```python
from build123d import *

# Parameters (mm, degrees)
SKETCH001_W     = 308.102
SKETCH001_H     = 147.6375
PAD_DEPTH       = 12.7
SKETCH002_W     = 292.1
SKETCH002_H     = 128.5875
POCKET_DEPTH    = 3.556
SKETCH_W        = 300.0375
SKETCH_H        = 134.9375
POCKET001_DEPTH = 1.778
SKETCH003_W     = 20.6375
SKETCH003_H     = 38.1
POCKET002_DEPTH = 7.9375
SKETCH004_W     = 107.95
SKETCH004_H     = 34.925
POCKET003_DEPTH = 3.175


with BuildPart() as part:
    # Sketch001 → Pad (new body)
    with BuildSketch(Plane.XY):
        Rectangle(SKETCH001_W, SKETCH001_H)
    extrude(amount=PAD_DEPTH)

    # Sketch002 → Pocket (cut)
    with BuildSketch(Plane.XY.offset(12.7)):
        Rectangle(SKETCH002_W, SKETCH002_H)
    extrude(amount=-POCKET_DEPTH, mode=Mode.SUBTRACT)

    # Sketch → Pocket001 (cut)
    with BuildSketch(Plane.XY.offset(12.7)):
        Rectangle(SKETCH_W, SKETCH_H)
    extrude(amount=-POCKET001_DEPTH, mode=Mode.SUBTRACT)

    # Sketch003 → Pocket002 (cut)
    with BuildSketch(Plane.XY.offset(10.922)):
        with Locations((0, 48.41875)):
            Rectangle(SKETCH003_W, SKETCH003_H)
    extrude(amount=-POCKET002_DEPTH, mode=Mode.SUBTRACT)

    # Sketch004 → Pocket003 (cut)
    with BuildSketch(Plane.XY.offset(9.144)):
        with Locations((-64.29375, 46.83125)):
            Rectangle(SKETCH004_W, SKETCH004_H)
    extrude(amount=-POCKET003_DEPTH, mode=Mode.SUBTRACT)


solid = part.part
```
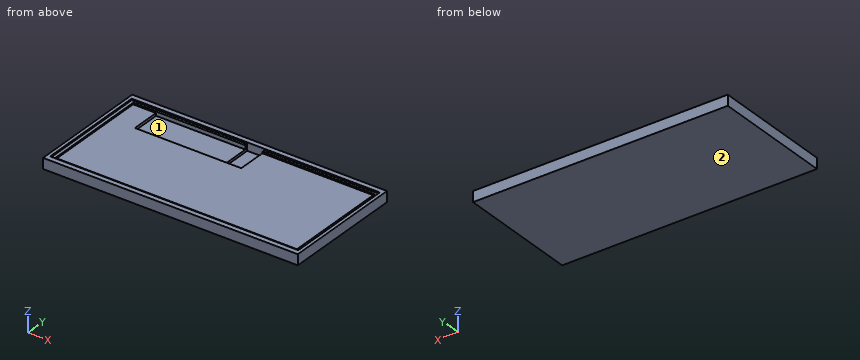
CAD build for the part. Positions are in the model's coordinates, mm. Face numbers are marked on the shaded views. Round coordinates to 2 decimals unless told otherwise and drop trailing zeros. Write each loop counter-clockwise with the first axis right and the second up, starting at its lowest first coordinate (ties: lowest second). Pieces come first, ordered by that corner, then holes. Notation, with made-up numbers: (65, 34) -> (74, 34) arc R11 cw to (74, 54) -> close; hole circle Ø5 at (80, 44.5). An arc over 180 degrees is marked (long way). Answer in a Markdown table with one row per item. Add a question column.
Item 1: Saw through at A-A, the plane x = -4.5. Write the cut outline in (y, z), then the cut area to 3 significant figures.
Item 2: Saw through at D-D, the plane x = -93. Write the cut outline in (y, z), then the cut area to 3 significant figures.
Item 3: Drop flat-ended pins along their axis: pin 1 Ø6 at (x, y) = (40, -8) entering from -Z; pin 2 Ø8 at (x, y) = (-81.5, 11.5) entering from +Z; pin 3 Ø6 at (x, y) = (-2.5, 40) entering from +Z. Give the stop position or say it passes through.
Item 4: Saw through at C-C, the plane x = 109.5. Write the cut outline in (y, z).
Item 5: Drill centre lines: line 1 (X direction, y = -49.5, z = 12.25); line 2 (X direction, y = -31.5, z = 9.75); line 3 (Y direction, x = -88, z = 8.25). Where is each one in solid material? Low to high. Write a range as from..to.
Item 6: Saw through at B-B, the plane y = 38.5. Write the cut outline in (x, z).
Item 7: Mould opens along X. For the marked faces 1 and 2 say: pulls with the +X half, pulls with the -X half, needs draft (parallel to the pull), parting line crosses it, or undercut.
Findings below:
| question | item | result |
|---|---|---|
| 1 | outline | (-73.82, 0) -> (73.82, 0) -> (73.82, 12.7) -> (67.47, 12.7) -> (67.47, 2.98) -> (29.37, 2.98) -> (29.37, 9.14) -> (-64.29, 9.14) -> (-64.29, 10.92) -> (-67.47, 10.92) -> (-67.47, 12.7) -> (-73.82, 12.7) -> close |
| 1 | area | 1,170 mm^2 |
| 2 | outline | (-73.82, 0) -> (73.82, 0) -> (73.82, 12.7) -> (67.47, 12.7) -> (67.47, 10.92) -> (64.29, 10.92) -> (64.29, 5.97) -> (29.37, 5.97) -> (29.37, 9.14) -> (-64.29, 9.14) -> (-64.29, 10.92) -> (-67.47, 10.92) -> (-67.47, 12.7) -> (-73.82, 12.7) -> close |
| 2 | area | 1,300 mm^2 |
| 3 | pin 1 | stops at z = 0 |
| 3 | pin 2 | stops at z = 9.14 |
| 3 | pin 3 | stops at z = 2.98 |
| 4 | outline | (-73.82, 0) -> (73.82, 0) -> (73.82, 12.7) -> (67.47, 12.7) -> (67.47, 10.92) -> (64.29, 10.92) -> (64.29, 9.14) -> (-64.29, 9.14) -> (-64.29, 10.92) -> (-67.47, 10.92) -> (-67.47, 12.7) -> (-73.82, 12.7) -> close |
| 5 | line 1 | x = -154.05..-150.02, 150.02..154.05 |
| 5 | line 2 | x = -154.05..-146.05, 146.05..154.05 |
| 5 | line 3 | y = -73.82..29.37, 64.29..73.82 |
| 6 | outline | (-154.05, 0) -> (154.05, 0) -> (154.05, 12.7) -> (150.02, 12.7) -> (150.02, 10.92) -> (146.05, 10.92) -> (146.05, 9.14) -> (10.32, 9.14) -> (10.32, 2.98) -> (-10.32, 2.98) -> (-10.32, 5.97) -> (-118.27, 5.97) -> (-118.27, 9.14) -> (-146.05, 9.14) -> (-146.05, 10.92) -> (-150.02, 10.92) -> (-150.02, 12.7) -> (-154.05, 12.7) -> close |
| 7 | face 1 | undercut |
| 7 | face 2 | needs draft |
